Autodesk Inventor part; units mm, degrees
ref_plane "YZ Plane" through (0, 0, 0) normal (1, 0, 0) x (0, 1, 0)
ref_plane "XZ Plane" through (0, 0, 0) normal (0, 1, 0) x (-1, 0, 0)
ref_plane "XY Plane" through (0, 0, 0) normal (0, 0, 1) x (1, 0, 0)
sketch "Sketch1" plane through (0, 0, 0) normal (0, 0, 1) x (1, 0, 0)
  line L0 (0, 0) -> (-5, 0)
  line L1 (-5, 0) -> (-5, -128.15)
  line L2 (-5, -128.15) -> (0, -128.15)
  line L3 (0, -128.15) -> (0, 0)
  line L4 (0, 0) -> (-13.1356, 0) construction
  dimension "d1" = 128.15
  dimension "d2" = 5
revolve "Shoulder" add sketch "Sketch1" angle 360 about axis through (0, -128.15, 0) along (0, 1, 0)
sketch "Sketch2" plane through (0, 0, 0) normal (0, 1, 0) x (1, 0, 0)
  circle A0 centre (0, 0) radius 5
  circle A1 centre (0, 0) radius 4.76
  dimension "d3" = 9.52
extrude "Shoulder_neck" add sketch "Sketch2" along normal blind 1.85 contours A1
sketch "Sketch3" plane through (0, 1.85, 0) normal (0, 1, 0) x (1, 0, 0)
  circle A0 centre (0, 0) radius 4.76
  circle A1 centre (0, 0) radius 8.1
  dimension "d6" = 16.2
extrude "Head" add sketch "Sketch3" along normal blind 7 contours A0 | A1
sketch "Sketch4" plane through (0, -128.15, 0) normal (0, -1, 0) x (1, 0, 0)
  circle A0 centre (0, 0) radius 5
  circle A1 centre (0, 0) radius 3.09
  dimension "d9" = 6.18
extrude "Thread_neck" add sketch "Sketch4" along normal blind 2.6 contours A1
sketch "Sketch5" plane through (0, -130.75, 0) normal (0, -1, 0) x (1, 0, 0)
  circle A0 centre (0, 0) radius 3.09
  circle A1 centre (0, 0) radius 4
  dimension "d12" = 8
extrude "Thread_shoulder" add sketch "Sketch5" along normal blind 10.4 contours A0 | A1
sketch "Sketch6" plane through (0, 8.85, 0) normal (0, 1, 0) x (1, 0, 0)
  circle A0 centre (0, 0) radius 8.1
  circle A1 centre (0, 0) radius 2.5 construction
  line L0 (-2.5, 1.4434) -> (-2.5, -1.4434)
  line L1 (-2.5, -1.4434) -> (0, -2.8868)
  line L2 (0, -2.8868) -> (2.5, -1.4434)
  line L3 (2.5, -1.4434) -> (2.5, 1.4434)
  line L4 (2.5, 1.4434) -> (0, 2.8868)
  line L5 (0, 2.8868) -> (-2.5, 1.4434)
  dimension "d15" = 5
extrude "Hex" cut sketch "Sketch6" against normal blind 4.2 contours L5 L4 L3 L2 L1 L0
chamfer "Chamfer1" distance 0.24 angle 30 1 edges at (5, 0, 0) measured on face at (-4.8255, 0, -0.7786)
fillet "Fillet1" radius 0.4 1 edges at (-4.76, 1.85, 0)
chamfer "Chamfer2" distance 0.5 angle 30 1 edges at (-8.1, 8.85, 0) measured on face at (7.9951, 6.5167, 1.2993)
chamfer "Chamfer3" distance 0.625 angle 30 1 edges at (-4, -141.15, 0) measured on face at (0.7574, -141.15, 1.0973)
fillet "Fillet2" radius 0.7 1 edges at (-3.09, -128.15, 0)
chamfer "Chamfer7" distance 0.91 angle 30 1 edges at (-4, -130.75, 0) measured on face at (3.6579, -130.75, -0.3191)
thread "Thread"
equation "\"d3\" = Shoulder_neck_dia"
equation "\"d4\" = Shoulder_neck_length"
equation "\"d6\" = Head_diameter"
equation "\"d7\" = Head_height"
equation "\"d9\" = Thread_neck_dia"
equation "\"d10\" = Thread_neck_length"
equation "\"d12\" = Thread_diameter"
equation "\"d13\" = Thread_length - Thread_neck_length"
equation "\"d15\" = Hex_size"
equation "\"d16\" = Hex_length"
equation "\"d18\" = -0.5 * Shoulder_neck_dia + 0.5 * Shoulder_diameter"
equation "\"d64\" = -0.5 * Shoulder_neck_dia + 0.5 * Shoulder_diameter"
equation "\"d21\" = 0.1 * Hex_size"
equation "\"d65\" = 0.1 * Hex_size"
equation "\"d23\" = 0.5 * Thread_pitch"
equation "\"d66\" = 0.5 * Thread_pitch"
equation "\"d25\" = Thread_neck_radius"
equation "\"d60\" = -0.5 * Thread_neck_dia + 0.5 * Thread_diameter"
equation "\"d67\" = -0.5 * Thread_neck_dia + 0.5 * Thread_diameter"
equation "\"d1\" = Shoulder_length - Shoulder_neck_length"
equation "\"d2\" = 0.5 * Shoulder_diameter"
equation "\"Shoulder_length\" = 130"
equation "\"Shoulder_neck_dia\" = 9.52"
equation "\"Thread_diameter\" = 8"
equation "\"Thread_length\" = 13"
equation "\"Head_diameter\" = 16.2"
equation "\"Head_height\" = 7"
equation "\"Thread_neck_dia\" = 6.18"
equation "\"Hex_size\" = 5"
equation "\"Hex_length\" = 4.2"
equation "\"Thread_pitch\" = 1.25"
equation "\"Shoulder_neck_length\" = 1.85"
equation "\"Thread_neck_length\" = 2.6"
equation "\"Thread_neck_radius\" = 0.7"
properties part number "SCREW,SHOULDER,P,12.9,M10X130MM" material "Steel, High Strength Low Alloy"
Here's how the part is built. I have some questions about the finished solid (model axes, mm). A direction names the side the tool comes from. Coordinates: 2 decimals unless noted, no trailing zeros. Order: outer loops, then holes, each group sorted by start corner. A loop starts at its lowest first (then second) coordinate and runs counter-clockwise, first axis right, second up. Notation, with made-up numbers: (59, -22.75) - (96, -22.75) arc R21 cw to (96, -15.75) - close; hole circle Ø6 at (16, -37.75). An arc over 180 degrees is marked (long way). Use CSV: the item, a comma, the result in double quotes. Start each with the question number.
1. Suppose I cut it at A-A on y = -14.5. List the corners of the cut face in (x, z) for me.
2. If we mould it in two halves opening along Z, with no side actions, what happens to faces 5 (the face through (-1.032, 0.715, -4.647)), 6 (the face through (5, 1.85, 2)), 7 (the face through (1.267, 6.779, -2.155)), 8 (the face through (2.5, 7, 0))? For each: +Z half, -Z half, draft (parallel to the pull), parting line (faces both ways), or undercut.
3. For faces 1 (the face through (0, -141.15, 0)), 2 (the face through (1.08, -65.04, 4.88)), 3 (the face through (1.233, 6.779, 2.175)), 4 (the face through (1.661, -129.787, -2.605)), which set-ups out of +Z, -Z, +X, -X, +Y, -Y let a thin tool reach every point of the face, with its end or its side?
4. I'm going to push flat-ended pins straight in: pin 1 (8 mm diameter, centred on y = -22.5, z = 3.5, fed in from +X); pin 2 (4 mm diameter, centred on x = 2, y = -101.5, fed in from +Z); pin 3 (5 mm diameter, centred on y = -48.5, z = 2.5, fed in from -X); pin 4 (1 mm diameter, centred on x = 6, z = -6.5, fed in from -Y). Where does each tip first touch, or does it pass through?
5. Please list where these lines run through material, in increasing order: line 1 (X direction, y = -27.5, z = -0.25); line 2 (Y direction, x = 0.75, z = -0.25); line 3 (X direction, y = -27.5, z = 3). Write a range as from..to.
Output:
1,outline,"circle Ø10 at (0, 0)"
2,face 5,"parting line"
2,face 6,"draft"
2,face 7,"undercut"
2,face 8,"undercut"
3,face 1,"+Z, -Z, +X, -X, -Y"
3,face 2,"-Y"
3,face 3,"+Y"
3,face 4,"none"
4,pin 1,"stops at x = 5"
4,pin 2,"stops at z = 5"
4,pin 3,"stops at x = -5"
4,pin 4,"passes through"
5,line 1,"x = -4.99..4.99"
5,line 2,"y = -141.15..4.65"
5,line 3,"x = -4..4"
